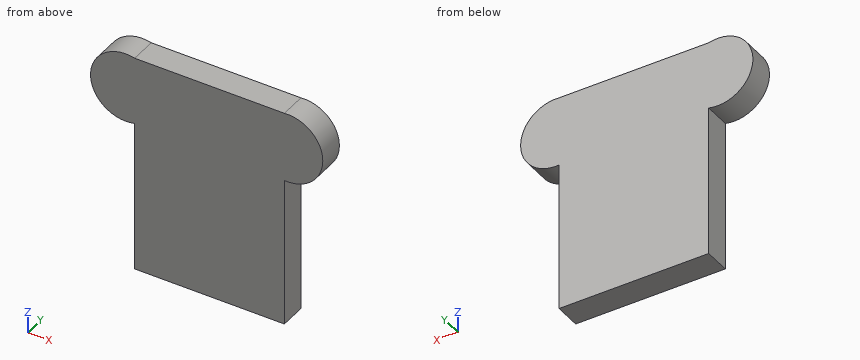
```python
from build123d import *

# Parameters (mm, degrees)
F1_DEPTH = 3


with BuildPart() as f1:
    # F0 (on Front) → F1 (new body)
    with BuildSketch(Plane.XZ):
        with BuildLine():
            ThreePointArc((-2.900381, 19.007138), (-7.917083, 15.138505), (-2.900381, 11.269873))
            Line((-2.900381, 11.269873), (-2.900381, -5.992862))
            Line((-2.900381, -5.992862), (14.099619, -5.992862))
            Line((14.099619, -5.992862), (14.099619, 11.040998))
            ThreePointArc((14.099619, 11.040998), (18.467255, 15.024068), (14.099619, 19.007138))
            Line((14.099619, 19.007138), (-2.900381, 19.007138))
        make_face()
    extrude(amount=F1_DEPTH)


solid = f1.part
```
Check sheet for the modelled part. Datum: model origin and axes. Units: mm. Give positions to 0.01 mm unless a question says otherwise; leave off trailing zeros. Write each loop counter-clockwise with the first axis right and the second up, starting at its lowest first coordinate (ties: lowest second). Pieces come first, ordered by that corner, then holes. Notation, with made-up numbers: (-25.75, 48) -> (-11.75, 48) arc R15 ccw to (-11.75, 68) -> close; hole circle Ø2 at (61, -39). An arc over 180 degrees is marked (long way). Use CSV: the item, a comma, the result in double quotes. Start each with the question number.
Q1. Cross-section at A-A on y = -2.6. Enter the section's corners in (x, z).
Q2. Cross-section at B-B on z = 2. Enter the section's corners in (x, y), and give its area (3 significant figures).
Q3. Cross-section at C-C on x = 16. Enter the section's corners in (y, z), and give its area (3 significant figures).
Q4. Depth check by flat-ended pin: P1, Ø0.9, axis at y = -1, z = 6.5, coming from the +X side; P2, Ø1, axis at x = 0, y = -1.5, coming from the +Z side; P3, Ø1.5, axis at y = -1.5, z = 0, coming from the -X side. Enter the tip coordinate at first touch or a pass-through.
Q5. Scan lines: line 1 along Z through (x, y) = (-2.25, -0.1); line 2 along X through (y, z) = (-1.85, 6.75); line 3 along Z through (x, y) = (14.25, -2.7). Record each from-to range of solid material in increasing order.
Working result:
1,outline,"(-2.9, -5.99) -> (14.1, -5.99) -> (14.1, 11.04) arc R4 ccw (long way) to (14.1, 19.01) -> (-2.9, 19.01) arc R4 ccw (long way) to (-2.9, 11.27) -> close"
2,outline,"(-2.9, -3) -> (14.1, -3) -> (14.1, 0) -> (-2.9, 0) -> close"
2,area,"51.0 mm^2"
3,outline,"(-3, 11.33) -> (0, 11.33) -> (0, 18.72) -> (-3, 18.72) -> close"
3,area,"22.2 mm^2"
4,P1,"stops at x = 14.1"
4,P2,"stops at z = 19.01"
4,P3,"stops at x = -2.9"
5,line 1,"z = -5.99 to 19.01"
5,line 2,"x = -2.9 to 14.1"
5,line 3,"z = 11.03 to 19.02"
